Model file for the job. Use its own axes, mm. Face numbers are marked on the shaded views. A direction names the side the tool comes from. Give positions to 0.01 mm unless a question says otherwise; leave off trailing zeros. Write each loop counter-clockwise with the first axis right and the second up, starting at its lowest first coordinate (ties: lowest second). Pieces come first, ordered by that corner, then holes.
```python
from build123d import *
from build123d.topology import SkipClean

# Parameters (mm, degrees)
SKETCH2_W               = 14
SKETCH2_H               = 6
BOSS_EXTRUDE1_DEPTH     = 4
SKETCH3_W               = 4
SKETCH3_H               = 6
BOSS_EXTRUDE2_DEPTH     = 12
CUT_EXTRUDE1_DEPTH      = 22.470910554
CUT_EXTRUDE1_DEPTH_BACK = 22.470910554
SKETCH4_R               = 1.5
BOSS_EXTRUDE3_START     = 1
SKETCH5_R               = 2.5
SKETCH5_R_2             = 1.5
BOSS_EXTRUDE3_DEPTH     = 1
SKETCH6_R               = 2.5
SKETCH6_R_2             = 1.5
BOSS_EXTRUDE4_DEPTH     = 1
SKETCH7_R               = 1
SKETCH7_W               = 4
SKETCH7_H               = 6
BOSS_EXTRUDE5_DEPTH     = 4
FILLET1_R               = 2
FILLET2_R               = 3


with BuildPart() as part:
    # Sketch2 → Boss-Extrude1 (new body)
    with BuildSketch(Plane(origin=(0, 0, 0), x_dir=(1, 0, 0), z_dir=(0, 1, 0))):
        Rectangle(SKETCH2_W, SKETCH2_H)
    extrude(amount=BOSS_EXTRUDE1_DEPTH)

    # Sketch3 → Boss-Extrude2 (add)
    with BuildSketch(Plane(origin=(0, 4, 0), x_dir=(1, 0, 0), z_dir=(0, 1, 0))):
        with Locations((-5, 0)):
            Rectangle(SKETCH3_W, SKETCH3_H)
        with Locations((5, 0)):
            Rectangle(SKETCH3_W, SKETCH3_H)
    extrude(amount=BOSS_EXTRUDE2_DEPTH)

    # Sketch4 → Cut-Extrude1 (cut, two sides: drawn at the far end of the back side and taken through both)
    with BuildSketch(Plane(origin=(7, 0, 0), x_dir=(0, 0, -1), z_dir=(1, 0, 0)).offset(-CUT_EXTRUDE1_DEPTH_BACK)):
        with Locations((0, 12)):
            Circle(SKETCH4_R)
    extrude(amount=CUT_EXTRUDE1_DEPTH + CUT_EXTRUDE1_DEPTH_BACK, mode=Mode.SUBTRACT)

    # Sketch5 → Boss-Extrude3 (add)
    with BuildSketch(Plane(origin=(-3, 0, 0), x_dir=(0, 0, -1), z_dir=(1, 0, 0)).offset(BOSS_EXTRUDE3_START)):
        with Locations(Location((0, 12, 0), (0, 0, 180))):
            Circle(SKETCH5_R)
        with Locations((0, 12)):
            Circle(SKETCH5_R_2, mode=Mode.SUBTRACT)
    extrude(amount=-BOSS_EXTRUDE3_DEPTH)

    # Sketch6 → Boss-Extrude4 (add)
    with SkipClean():  # the faces are left unmerged after this step: merging them gives an invalid solid
        with BuildSketch(Plane.ZY.offset(-3)):
            with Locations((0, 12)):
                Circle(SKETCH6_R)
            with Locations((0, 12)):
                Circle(SKETCH6_R_2, mode=Mode.SUBTRACT)
        extrude(amount=BOSS_EXTRUDE4_DEPTH)

    # Sketch7 → Boss-Extrude5 (add)
    # profile 1 of 2: a face of its own
    with SkipClean():  # the faces are left unmerged after this step: merging them gives an invalid solid
        with BuildSketch(Plane(origin=(0, 4, 0), x_dir=(1, 0, 0), z_dir=(0, 1, 0))):
            Polygon((11, 3), (11, -3), (11, -11), (7, -11), (7, -3), (7, 3), align=None)
            with Locations(Location((9, -8, 0), (0, 0, 270))):
                Circle(SKETCH7_R, mode=Mode.SUBTRACT)
        # profile 2 of 2: a face of its own
        with BuildSketch(Plane(origin=(0, 4, 0), x_dir=(1, 0, 0), z_dir=(0, 1, 0))):
            with Locations((-9, 0)):
                Rectangle(SKETCH7_W, SKETCH7_H)
            with Locations(Location((-9, 0, 0), (0, 0, 270))):
                Circle(SKETCH7_R, mode=Mode.SUBTRACT)
        extrude(amount=-BOSS_EXTRUDE5_DEPTH)

    # Fillet1
    fillet1_edges = [part.edges().sort_by_distance(p)[0] for p in [
        (-11, 2, -3),
        (11, 2, -3),
        (11, 2, 11),
        (7, 2, 11),
        (-11, 2, 3),
        (7, 2, 3),
    ]]
    fillet(fillet1_edges, radius=FILLET1_R - 0.0001)  # a hair under: the kernel refuses the full size

    # Fillet2
    fillet2_edges = [part.edges().sort_by_distance(p)[0] for p in [
        (-5, 16, -3),
        (5, 16, -3),
        (5, 16, 3),
        (-5, 16, 3),
    ]]
    fillet(fillet2_edges, radius=FILLET2_R - 0.0001)  # a hair under: the kernel refuses the full size


solid = part.part
```
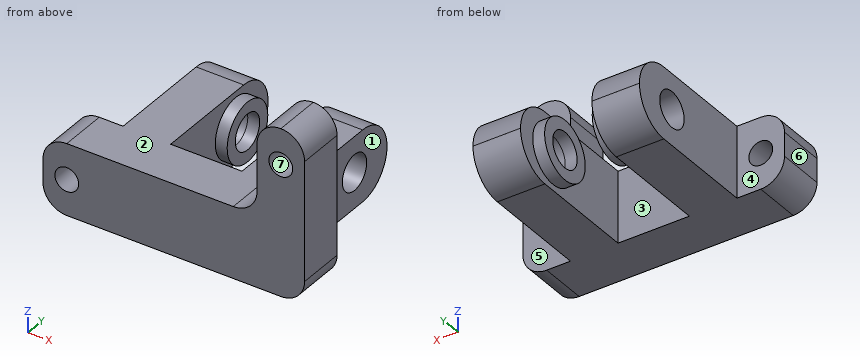
1. Slice it at B-B, the plane z = 0.75. State how many separate pieces and enclosed holes the cut face has, and give its area (3 significant figures).
Calculated:
separate pieces: 4
enclosed holes: 0
area: 162 mm2
2. Which spindle directions (+Z, -Z, +X, -X, +Y, -Y) get a long thin tool onto all of the face, cutting with end or side? Do the marked faces 1, 2, 3 and 4. Say none if no direction does.
Calculated:
face 1: +Z, -Z, +X, +Y
face 2: +Z, -X, +Y
face 3: +Z, -Z
face 4: +Z, -Z, -X, +Y
3. Slice it at D-D, the plane y = 10.25. Write the cut outline in (x, z).
Calculated:
outline: (-7, -3) - (-3, -3) - (-3, -1.79) - (-2, -1.79) - (-2, 1.79) - (-3, 1.79) - (-3, 3) - (-7, 3) - close; (2, -1.79) - (3, -1.79) - (3, -3) - (7, -3) - (7, 3) - (3, 3) - (3, 1.79) - (2, 1.79) - close
4. Probe probe 1 along Y at (x, z) = (2.5, 0); probe 2 along Z at (x, y) = (-4.6, 12); probe 3 along X at (y, z) = (10.25, 1.25). List the from-to ranges inside material, lowest first.
Calculated:
probe 1: y = 0 to 4, 9.5 to 10.5, 13.5 to 14.5
probe 2: z = -3 to -1.5, 1.5 to 3
probe 3: x = -7 to -2, 2 to 7
5. Pull direction X, two halves, no side cores. Call the marked faces 5, 6 and 7: +X half, -X half, draft (parallel to the pull), parting line (faces both ways), or undercut.
Calculated:
face 5: draft
face 6: -X half
face 7: undercut
6. Slice it at A-A, the plane y = 12. Write the cut outline in (x, z).
Calculated:
outline: (-7, -3) - (-3, -3) - (-3, -2.5) - (-2, -2.5) - (-2, -1.5) - (-7, -1.5) - close; (-7, 1.5) - (-2, 1.5) - (-2, 2.5) - (-3, 2.5) - (-3, 3) - (-7, 3) - close; (2, -2.5) - (3, -2.5) - (3, -3) - (7, -3) - (7, -1.5) - (2, -1.5) - close; (2, 1.5) - (7, 1.5) - (7, 3) - (3, 3) - (3, 2.5) - (2, 2.5) - close
7. Pin check, flat tips, straight feed: P1, Ø1.8, axis at y = 12.5, z = -1, coming from the +X side; P2, Ø3.5, axis at y = 12, z = 0, coming from the -X side; P3, Ø8, axis at x = -2.5, z = 9.5, coming from the +Y side; P4, Ø5, axis at x = 7, z = 5, coming from the +Y side. Stop position of each tip, or through.
Calculated:
P1: stops at x = 7
P2: stops at x = -7
P3: passes through
P4: stops at y = 14.66
